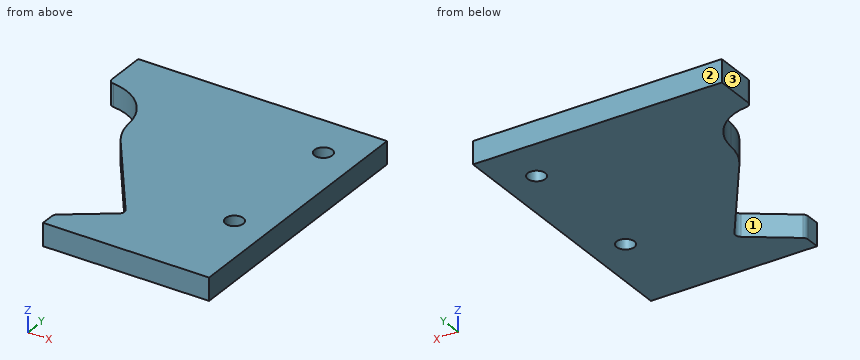
from build123d import *

# Parameters (mm, degrees)
SKETCH1_R           = 2.4892
BOSS_EXTRUDE1_DEPTH = 3.175
FILLET1_R           = 1.5875


with BuildPart() as part:
    # Sketch1 → Boss-Extrude1 (new, symmetric)
    with BuildSketch(Plane.XY):
        with BuildLine():
            Line((23.229645255, -44.228270645), (37.052935248, -34.429965394))
            Line((37.052935248, -34.429965394), (17.517315641, -6.869430374))
            ThreePointArc((17.517315641, -6.869430374), (15.535368252, -3.075379389), (14.639156809, 1.110279863))
            ThreePointArc((14.639156809, 1.110279863), (9.980916609, 10.766565705), (0, 14.6812))
            Line((0, 14.6812), (0, 27.3812))
            Line((0, 27.3812), (69.85, 27.3812))
            Line((69.85, 27.3812), (69.85, -48.8188))
            Line((69.85, -48.8188), (23.229645255, -48.8188))
            Line((23.229645255, -48.8188), (23.229645255, -44.228270645))
        make_face()
        with Locations((60.325, 14.6812)):
            Circle(SKETCH1_R, mode=Mode.SUBTRACT)
        with Locations((60.325, -23.4188)):
            Circle(SKETCH1_R, mode=Mode.SUBTRACT)
    extrude(amount=BOSS_EXTRUDE1_DEPTH, both=True)

    # Fillet1
    fillet1_edges = [part.edges().sort_by_distance(p)[0] for p in [
        (0, 14.6812, 0),
        (23.229645255, -44.228270645, 0),
        (37.052935248, -34.429965394, 0),
    ]]
    fillet(fillet1_edges, radius=FILLET1_R)


solid = part.part
Source: CAD feature listing. Evaluate the final solid. Frame: model axes, mm. Face numbers are marked on the shaded views. Round coordinates to 2 decimals unless told otherwise and drop trailing zeros. Loops run counter-clockwise (first coordinate to the right, second up) from the corner with the lowest first, then second, coordinate; pieces in that order, holes last.
Q1. Section B-B, the plane x = 60. Return loops of the section in (y, z) (3 decimals), plus the area to 3 significant figures.
Q2. Section C-C, the plane z = -2.25. State how many separate pieces and enclosed holes the cut face has, plus the area to 3 significant figures.
Q3. Ray query, line 1 (Y direction, x = 59.5, z = 0); line 2 (X direction, y = -24, z = -0.5); line 3 (X direction, y = -45, z = 0.75). Return the intervals inside material, ascending.
Q4. Mould query, pull axis Y, two halves, no side actions, for the marked faces 1, 2 and 3. Classes: pulls with the +Y half, pulls with the -Y half, needs draft (parallel to the pull), parting line crosses it, or undercut.
Q5. Section A-A, the plane x = 31. Return loops of the section in (y, z) (3 decimals), plus the area to 3 significant figures.
Q6. First-contact query: P1, Ø5.5, axis at x = 60.32, y = 14.68, coming from the -Z side (3 decimals); P2, Ø4.5, axis at x = 60.32, y = -23.42, coming from the +Z side. Flat tips, straight axial feed; report the tip coordinate or a pass-through.
Q7. Section D-D, the plane y = -13.5. Return loops of the section in (x, z) (3 decimals), plus the area to 3 significant figures.
Solutions:
1. outline: (-48.819, -3.175) - (-25.887, -3.175) - (-25.887, 3.175) - (-48.819, 3.175) - close; (-20.951, -3.175) - (12.213, -3.175) - (12.213, 3.175) - (-20.951, 3.175) - close; (17.149, -3.175) - (27.381, -3.175) - (27.381, 3.175) - (17.149, 3.175) - close
1. area: 421 mm2
2. separate pieces: 1
2. enclosed holes: 2
2. area: 3,850 mm2
3. line 1: y = -48.82 to -25.77, -21.07 to 12.33, 17.03 to 27.38
3. line 2: x = 29.66 to 57.9, 62.75 to 69.85
3. line 3: x = 23.23 to 69.85
4. face 1: undercut
4. face 2: pulls with the +Y half
4. face 3: needs draft
5. outline: (-48.819, -3.175) - (-38.72, -3.175) - (-38.72, 3.175) - (-48.819, 3.175) - close; (-25.891, -3.175) - (27.381, -3.175) - (27.381, 3.175) - (-25.891, 3.175) - close
5. area: 402 mm2
6. P1: stops at z = -3.175
6. P2: passes through
7. outline: (22.217, -3.175) - (69.85, -3.175) - (69.85, 3.175) - (22.217, 3.175) - close
7. area: 302 mm2
